Could you check a few things on this model? Use its own coordinates, in mm. A direction names the side the tool comes from. Round coordinates to 2 decimals unless told otherwise and drop trailing zeros. Write each loop counter-clockwise with the first axis right and the second up, starting at its lowest first coordinate (ties: lowest second). Pieces come first, ordered by that corner, then holes. Notation, with made-up numbers: (26.25, 20.5) -> (79.25, 20.5) arc R12 ccw to (79.25, 36.5) -> close; hole circle Ø7 at (-27.5, 26.25). An arc over 180 degrees is marked (long way). Return JSON: item names as keys, results as strings.
Autodesk Inventor part; units mm, degrees
ref_plane "YZ Plane" through (0, 0, 0) normal (1, 0, 0) x (0, 1, 0)
ref_plane "XZ Plane" through (0, 0, 0) normal (0, 1, 0) x (-1, 0, 0)
ref_plane "XY Plane" through (0, 0, 0) normal (0, 0, 1) x (1, 0, 0)
sketch "Skizze1" plane through (0, 0, 0) normal (0, 1, 0) x (-1, 0, 0)
  arc A0 (-7.5, 0) -> (7.5, 0) centre (0, 0) ccw
  line L0 (-14, 14) -> (-14, -14)
  line L1 (-14, -14) -> (14, -14)
  line L2 (14, -14) -> (14, 14)
  line L3 (7.5, 0) -> (7.5, 14)
  line L4 (-7.5, 0) -> (-7.5, 14)
  line L5 (14, 14) -> (7.5, 14)
  line L6 (-7.5, 14) -> (-14, 14)
  dimension "d0" = 15
  dimension "d1" = 28
  dimension "d2" = 28
  dimension "d3" = 14
  dimension "d4" = 14
extrude "Extrusion1" add sketch "Skizze1" against normal blind 49.5
sketch "Skizze2" plane through (0, -49.5, 0) normal (0, -1, 0) x (1, 0, 0)
  line L0 (-14, 14) -> (-14, -14)
  line L1 (-14, -14) -> (14, -14)
  line L2 (14, -14) -> (14, 14)
  line L3 (14, 14) -> (7.5, 14)
  line L4 (7.5, 14) -> (7.5, 0)
  arc A0 (-7.5, 0) -> (7.5, 0) centre (0, 0) ccw
  line L5 (-7.5, 0) -> (-7.5, 14)
  line L6 (-7.5, 14) -> (-14, 14)
  line L7 (-7.5, 0) -> (-7.5, 14)
  line L8 (-7.5, 14) -> (7.5, 14)
  circle A1 centre (0, 0) radius 5.2
  dimension "d7" = 10.4
extrude "Extrusion2" add sketch "Skizze2" against normal blind 5 contours L8 L4 A0 L5
chamfer "Fase1" distance 2.25 angle 45 1 edges at (-5.2, -44.5, 0)
sketch "Skizze5" plane through (0, 0, 0) normal (0, 1, 0) x (1, 0, 0)
  circle A0 centre (-11.5, -11.5) radius 1.25
  line L0 (-14, -14) -> (-14, 14)
  line L1 (-7.5, -14) -> (-14, -14)
  line L2 (-7.5, 0) -> (-7.5, -14)
  arc A1 (7.5, 0) -> (-7.5, 0) centre (0, 0) ccw
  line L3 (7.5, -14) -> (7.5, 0)
  line L4 (14, -14) -> (7.5, -14)
  line L5 (14, 14) -> (14, -14)
  line L6 (-14, 14) -> (14, 14)
  circle A2 centre (11.5, -11.5) radius 1.25
  circle A3 centre (-11.5, 11.5) radius 1.25
  circle A4 centre (11.5, 11.5) radius 1.25
  dimension "d21" = 2.5
  dimension "d22" = 2.5
  dimension "d23" = 2.5
  dimension "d26" = 23
  dimension "d29" = 23
extrude "Extrusion5" cut sketch "Skizze5" against normal blind 50 contours A0 | A2 | A3 | A4
sketch "Skizze7" plane through (0, -49.5, 0) normal (0, -1, 0) x (1, 0, 0)
  circle A0 centre (-11.5, 11.5) radius 1.25
  circle A1 centre (0, 0) radius 5.2
  line L0 (-14, 14) -> (-14, -14)
  line L1 (-14, -14) -> (14, -14)
  line L2 (14, -14) -> (14, 14)
  line L3 (14, 14) -> (-14, 14)
  circle A2 centre (11.5, 11.5) radius 1.25
  circle A3 centre (11.5, -11.5) radius 1.25
  circle A4 centre (-11.5, -11.5) radius 1.25
  line L4 (14, -14) -> (14, 14)
  line L5 (14, 14) -> (9, 14)
  line L6 (9, 14) -> (9, 9)
  line L7 (9, 9) -> (14, 9)
  line L8 (14, 9) -> (14, 14)
  line L9 (-14, 14) -> (-9, 14)
  line L10 (-9, 14) -> (-9, 9)
  line L11 (-9, 9) -> (-14, 9)
  line L12 (-14, 9) -> (-14, 14)
  line L13 (-14, -14) -> (-9, -14)
  line L14 (-9, -14) -> (-9, -9)
  line L15 (-9, -9) -> (-14, -9)
  line L16 (-14, -9) -> (-14, -14)
  line L17 (14, -14) -> (9, -14)
  line L18 (9, -14) -> (9, -9)
  line L19 (9, -9) -> (14, -9)
  line L20 (14, -9) -> (14, -14)
  line L21 (9, 9) -> (-9, 9)
  line L22 (-9, 9) -> (-9, 14)
  line L23 (-9, 14) -> (9, 14)
  line L24 (9, 14) -> (9, 9)
  dimension "d45" = 5
  dimension "d46" = 5
  dimension "d47" = 5
  dimension "d48" = 5
  dimension "d49" = 5
  dimension "d50" = 5
extrude "Extrusion7" cut sketch "Skizze7" against normal blind 40.5 contours A0 | L3 L10 L11 L0 | L3 L6 L21 L10 | L15 L14 L1 L0 | L3 L2 L7 L6 | L18 L19 L2 L1 | A2 | A3 | A4
fillet "Rundung3" radius 2 6 edges at (14, -29.25, 9) (14, -29.25, -9) (-14, -29.25, 9) (9, -29.25, -14) (-9, -29.25, -14) (-14, -29.25, -9)
sketch "Skizze8" plane through (0, -49.5, 0) normal (0, -1, 0) x (1, 0, 0)
  circle A0 centre (0, 0) radius 5.2
  arc A1 (-14, -7) -> (-12, -9) centre (-12, -7) ccw
  line L0 (-12, -9) -> (-9, -9)
  line L1 (-9, -9) -> (-9, -12)
  arc A2 (-9, -12) -> (-7, -14) centre (-7, -12) ccw
  line L2 (-7, -14) -> (7, -14)
  arc A3 (7, -14) -> (9, -12) centre (7, -12) ccw
  line L3 (9, -12) -> (9, -9)
  line L4 (9, -9) -> (12, -9)
  arc A4 (12, -9) -> (14, -7) centre (12, -7) ccw
  line L5 (14, -7) -> (14, 7)
  arc A5 (14, 7) -> (12, 9) centre (12, 7) ccw
  line L6 (12, 9) -> (-12, 9)
  arc A6 (-12, 9) -> (-14, 7) centre (-12, 7) ccw
  line L7 (-14, 7) -> (-14, -7)
extrude "Extrusion8" cut sketch "Skizze8" against normal blind 1.5
properties part number "Lower_Unit"
1) I want a section at B-B, the plane x = 11.5. Please give me the cut outline in (y, z), and give its area (3 significant figures).
Return value:
{"outline": "(-48, -9) -> (-9, -9) -> (-9, -10.25) -> (0, -10.25) -> (0, 10.25) -> (-9, 10.25) -> (-9, 9) -> (-48, 9) -> close; (-9, -14) -> (0, -14) -> (0, -12.75) -> (-9, -12.75) -> close; (-9, 12.75) -> (0, 12.75) -> (0, 14) -> (-9, 14) -> close", "area": "909 mm²"}
2) I want a section at A-A, the plane z = -11.5. Please give me the cut outline in (x, y).
Return value:
{"outline": "(-14, -9) -> (-12.75, -9) -> (-12.75, 0) -> (-14, 0) -> close; (-10.25, -9) -> (-9, -9) -> (-9, -48) -> (9, -48) -> (9, -9) -> (10.25, -9) -> (10.25, 0) -> (-10.25, 0) -> close; (12.75, -9) -> (14, -9) -> (14, 0) -> (12.75, 0) -> close"}
3) For faces 1 (the face through (13, -9, -11)), 2 (the face through (-13, -9, -11)), 3 (the face through (-7.5, -22, 5)), which set-ups out of +Z, -Z, +X, -X, +Y, -Y let a thin tool reach every point of the face, with its end or its side?
Return value:
{"face 1": "-Z, +X, -Y", "face 2": "-Z, -X, -Y", "face 3": "+Z, +Y"}
4) I want a section at C-C, the plane z = 11.5. Please give me the cut outline in (x, y).
Return value:
{"outline": "(-14, -9) -> (-12.75, -9) -> (-12.75, 0) -> (-14, 0) -> close; (-10.25, -9) -> (-7.5, -9) -> (-7.5, 0) -> (-10.25, 0) -> close; (7.5, -9) -> (10.25, -9) -> (10.25, 0) -> (7.5, 0) -> close; (12.75, -9) -> (14, -9) -> (14, 0) -> (12.75, 0) -> close"}
5) Thinking about a two-plate mould opening in Z: for faces 4 (the face through (10, -29, -9)), 5 (the face through (9, -29, -11)), 6 (the face through (-12.421, -4.437, 10.655)), 7 (the face through (11, -4, 14)), which applies, pulls with the +Z half, pulls with the -Z half, needs draft (parallel to the pull), parting line crosses it, or undercut?
Return value:
{"face 4": "pulls with the -Z half", "face 5": "needs draft", "face 6": "undercut", "face 7": "pulls with the +Z half"}
6) If I drill on probe 1 along X at (y, z) = (-4.25, 11.5); probe 2 along Z at (x, y) = (-11.5, -2.5), over which ranges is the centre line in solid material (lowest first)? Write a range as [from, to].
Return value:
{"probe 1": "[-14, -12.75], [-10.25, -7.5], [7.5, 10.25], [12.75, 14]", "probe 2": "[-14, -12.75], [-10.25, 10.25], [12.75, 14]"}
7) Will these pins go through, and if not, where does the flat tip stop? pin 1 Ø3.5 at (y, z) = (-36.5, -10) entering from +X; pin 2 Ø4 at (y, z) = (-13.5, 9) entering from +X; pin 3 Ø0.9 at (x, y) = (-11, -33) entering from -Z; pin 4 Ø3.5 at (y, z) = (-29, -10.5) entering from -X.
Return value:
{"pin 1": "x = 13.56", "pin 2": "x = 14", "pin 3": "z = -9", "pin 4": "x = -12.97"}
8) I want a section at D-D, the plane x = 0. Please give me the cut outline in (y, z), and give its area (3 significant figures).
Return value:
{"outline": "(-48, -14) -> (0, -14) -> (0, -7.5) -> (-44.5, -7.5) -> (-44.5, -7.45) -> (-46.75, -5.2) -> (-48, -5.2) -> close; (-48, 5.2) -> (-46.75, 5.2) -> (-44.5, 7.45) -> (-44.5, 9) -> (-48, 9) -> close", "area": "328 mm²"}
